Geometry check sheet. Reference: drawing and pictorial views, mm from the part's lowest x, y, z. Give positions to 0.01 mm unless a question says otherwise; leave off trailing zeros. Write each loop counter-clockwise with the first axis right and the second up, starting at its lowest first coordinate (ties: lowest second). Pieces come first, ordered by that corner, then holes. Notation, with made-up numbers: (-36.75, 19) - (21.25, 19) arc R26 cw to (21.25, 37) - close; hole circle Ø5 at (-18, 37.25). An arc over 180 degrees is marked (long way). Put each result on its own line as item: value.
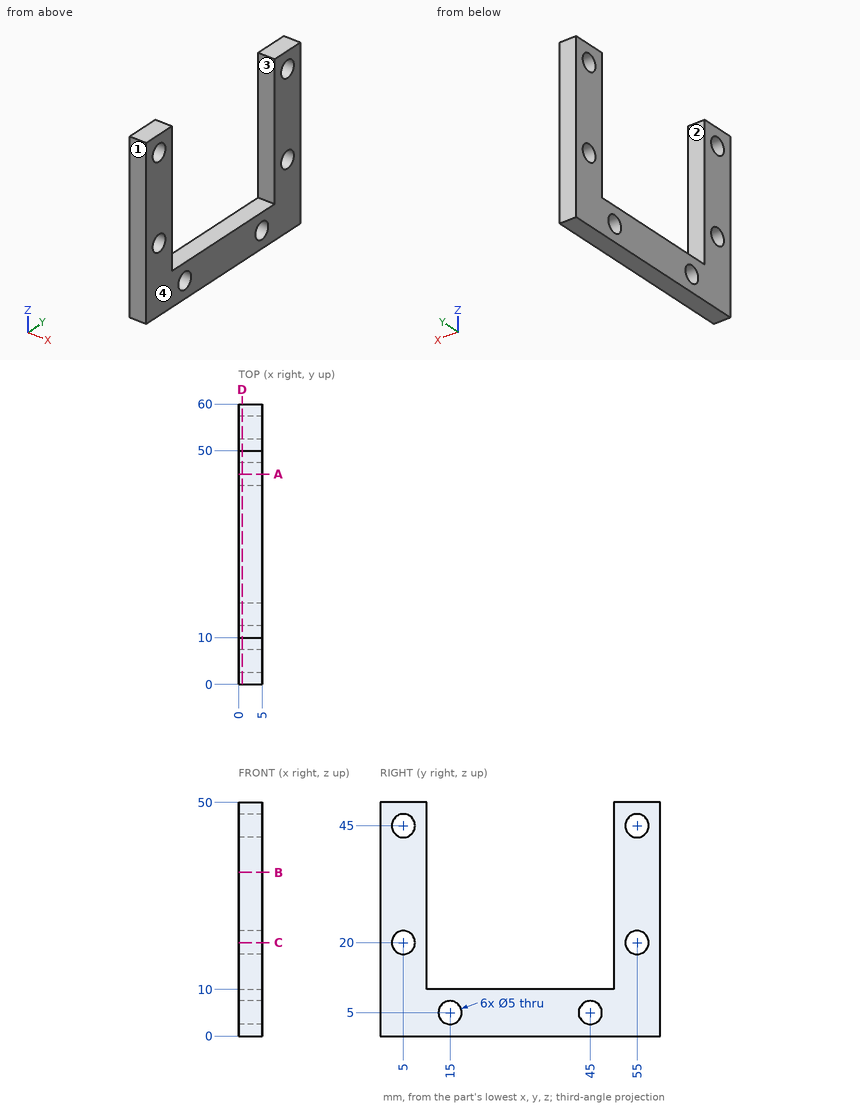
Q1. Section check D-D, the plane x = 0.75. Record the cut outline in (y, z), plus the area to 3 significant figures.
Answers follow:
outline: (0, 0) - (60, 0) - (60, 50) - (50, 50) - (50, 10) - (10, 10) - (10, 50) - (0, 50) - close; hole circle Ø5 at (5, 20); hole circle Ø5 at (5, 45); hole circle Ø5 at (15, 5); hole circle Ø5 at (45, 5); hole circle Ø5 at (55, 20); hole circle Ø5 at (55, 45)
area: 1,280 mm2
Q2. Section check C-C, the plane z = 20. Record the cut outline in (x, y).
Answers follow:
outline: (0, 0) - (5, 0) - (5, 2.5) - (0, 2.5) - close; (0, 7.5) - (5, 7.5) - (5, 10) - (0, 10) - close; (0, 50) - (5, 50) - (5, 52.5) - (0, 52.5) - close; (0, 57.5) - (5, 57.5) - (5, 60) - (0, 60) - close
Q3. Scan lines: line 1 along Z through (x, y) = (2.65, 55); line 2 along Y through (x, z) = (1.95, 22); line 3 along Y through (x, z) = (0.55, 15.5). Record each from-to range of solid material in increasing order.
Answers follow:
line 1: z = 0 to 17.5, 22.5 to 42.5, 47.5 to 50
line 2: y = 0 to 3.5, 6.5 to 10, 50 to 53.5, 56.5 to 60
line 3: y = 0 to 10, 50 to 60
Q4. Go/stop test with a flat-tipped pin: pin 1 Ø1 at (x, y) = (2.5, 27.5) entering from +Z. Record where the tip stops, or that it passes through.
Answers follow:
pin 1: stops at z = 10
Q5. Release check for a two-part mould opening along Y. For the marked faces 1, 2, 3 and 4 record: released by +Y, released by -Y, zero draft, split by the parting line, or undercut.
Answers follow:
face 1: released by -Y
face 2: undercut
face 3: undercut
face 4: zero draft
Q6. Section check A-A, the plane y = 45. Record the cut outline in (x, z).
Answers follow:
outline: (0, 0) - (5, 0) - (5, 2.5) - (0, 2.5) - close; (0, 7.5) - (5, 7.5) - (5, 10) - (0, 10) - close
Q7. Section check B-B, the plane z = 35. Record the cut outline in (x, y), plus the area to 3 significant figures.
Answers follow:
outline: (0, 0) - (5, 0) - (5, 10) - (0, 10) - close; (0, 50) - (5, 50) - (5, 60) - (0, 60) - close
area: 100 mm2
